Source: CAD feature listing. Evaluate the final solid. Frame: model axes, mm. Face numbers are marked on the shaded views. Give positions to 0.01 mm unless a question says otherwise; leave off trailing zeros. Order: outer loops, then holes, each group sorted by start corner. A loop starts at its lowest first (then second) coordinate and runs counter-clockwise, first axis right, second up. Notation, with made-up numbers: M 4,-1 L 57,-1 A18 ccw 57,16 Z; hole C -32.5,-30 d1. An arc over 180 degrees is marked long. Return JSON: item names as keys, results as strings.
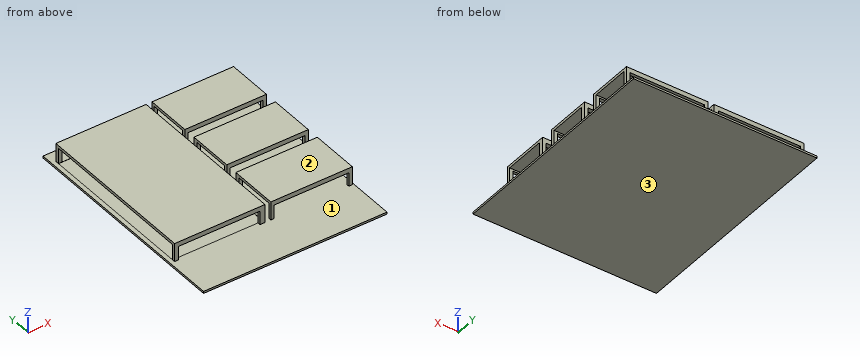
from build123d import *

# Parameters (mm, degrees)
SKETCH1_W               = 180
SKETCH1_H               = 220
BASE_DEPTH              = 2
SKETCH2_W               = 88.607017387
SKETCH2_H               = 162.747582956
SKETCH2_W_2             = 80
SKETCH2_H_2             = 45
SKETCH2_H_3             = 47.956874403
BOARDS_DEPTH            = 20
CUT_EXTRUDE1_DEPTH      = 285.956136976
CUT_EXTRUDE1_DEPTH_BACK = 285.956136976
SKETCH3_W               = 80.16842423
SKETCH3_H               = 13.497664936
SKETCH3_W_2             = 73.29684501
SKETCH4_W               = 15.397369521
SKETCH4_H               = 156.425076719
CUT_EXTRUDE2_DEPTH      = 88.607017387
SKETCH5_W               = 15.24584824
SKETCH5_H               = 38.4651821
SKETCH5_H_2             = 37.437486396
SKETCH5_H_3             = 40.814200855
CUT_EXTRUDE3_DEPTH      = 80


with BuildPart() as part:
    # Sketch1 → Base (new body)
    with BuildSketch(Plane.XY):
        with Locations((90, 110)):
            Rectangle(SKETCH1_W, SKETCH1_H)
    extrude(amount=BASE_DEPTH)

    # Sketch2 → Boards (add)
    with BuildSketch(Plane.XY):
        with Locations((48.5089102, 126.904245713)):
            Rectangle(SKETCH2_W, SKETCH2_H)
        with Locations((138.596199401, 185.778037191)):
            Rectangle(SKETCH2_W_2, SKETCH2_H_2)
        with Locations((138.596199401, 128.382682915)):
            Rectangle(SKETCH2_W_2, SKETCH2_H_2)
        with Locations((138.596199401, 69.508891437)):
            Rectangle(SKETCH2_W_2, SKETCH2_H_3)
    extrude(amount=BOARDS_DEPTH)

    # Sketch3 → Cut-Extrude1 (cut, two sides: drawn at the far end of the back side and taken through both)
    with BuildSketch(Plane(origin=(0, 0, 0), x_dir=(1, 0, 0), z_dir=(0, 1, 0)).offset(-CUT_EXTRUDE1_DEPTH_BACK)):
        with Locations((48.029472021, -8.748832468)):
            Rectangle(SKETCH3_W, SKETCH3_H)
        with Locations((138.50526508, -8.748832468)):
            Rectangle(SKETCH3_W_2, SKETCH3_H)
    extrude(amount=CUT_EXTRUDE1_DEPTH + CUT_EXTRUDE1_DEPTH_BACK, mode=Mode.SUBTRACT)

    # Sketch4 → Cut-Extrude2 (cut)
    with BuildSketch(Plane(origin=(92.812418893, 0, 0), x_dir=(0, 0, -1), z_dir=(1, 0, 0))):
        with Locations((-9.547163479, 126.516271725)):
            Rectangle(SKETCH4_W, SKETCH4_H)
    extrude(amount=-CUT_EXTRUDE2_DEPTH, mode=Mode.SUBTRACT)

    # Sketch5 → Cut-Extrude3 (cut)
    with BuildSketch(Plane(origin=(178.596199401, 0, 0), x_dir=(0, 0, -1), z_dir=(1, 0, 0))):
        with Locations((-9.62292412, 186.029564078)):
            Rectangle(SKETCH5_W, SKETCH5_H)
        with Locations((-9.62292412, 127.817943074)):
            Rectangle(SKETCH5_W, SKETCH5_H_2)
        with Locations((-9.62292412, 68.578626366)):
            Rectangle(SKETCH5_W, SKETCH5_H_3)
    extrude(amount=-CUT_EXTRUDE3_DEPTH, mode=Mode.SUBTRACT)


solid = part.part
1. Section query B-B (y = 139). Return loops of the section in (x, z), then the cut area to 3 significant figures.
Evaluation:
{"outline": "M 0,0 L 180,0 L 180,2 L 92.81,2 L 92.81,1.85 L 4.21,1.85 L 4.21,2 L 0,2 Z; M 4.21,17.25 L 92.81,17.25 L 92.81,20 L 4.21,20 Z; M 98.6,17.25 L 178.6,17.25 L 178.6,20 L 98.6,20 Z", "area": "811 mm^2"}
2. Section query A-A (x = 154.5). Return loops of the section in (y, z).
Evaluation:
{"outline": "M 0,0 L 220,0 L 220,2 L 0,2 Z; M 45.53,15.5 L 48.17,15.5 L 48.17,17.25 L 88.99,17.25 L 88.99,15.5 L 93.49,15.5 L 93.49,20 L 45.53,20 Z; M 105.88,15.5 L 109.1,15.5 L 109.1,17.25 L 146.54,17.25 L 146.54,15.5 L 150.88,15.5 L 150.88,20 L 105.88,20 Z; M 163.28,15.5 L 166.8,15.5 L 166.8,17.25 L 205.26,17.25 L 205.26,15.5 L 208.28,15.5 L 208.28,20 L 163.28,20 Z"}
3. Ray query, probe 1 along Y at (x, z) = (147, 17.75); probe 2 along Y at (x, z) = (90.5, 13.75); probe 3 along Z at (x, y) = (152.5, 127.5). Return the intervals inside material, ascending.
Evaluation:
{"probe 1": "y = 45.53 to 93.49, 105.88 to 150.88, 163.28 to 208.28", "probe 2": "y = 45.53 to 48.3, 204.73 to 208.28", "probe 3": "z = 0 to 2, 17.25 to 20"}
4. Section query D-D (x = 58). Return loops of the section in (y, z), then the cut area to 3 significant figures.
Evaluation:
{"outline": "M 0,0 L 220,0 L 220,2 L 204.73,2 L 204.73,1.85 L 48.3,1.85 L 48.3,2 L 0,2 Z; M 45.53,15.5 L 48.3,15.5 L 48.3,17.25 L 204.73,17.25 L 204.73,15.5 L 208.28,15.5 L 208.28,20 L 45.53,20 Z", "area": "876 mm^2"}
5. Section query C-C (y = 96.5). Return loops of the section in (x, z), then the cut area to 3 significant figures.
Evaluation:
{"outline": "M 0,0 L 180,0 L 180,2 L 92.81,2 L 92.81,1.85 L 4.21,1.85 L 4.21,2 L 0,2 Z; M 4.21,17.25 L 92.81,17.25 L 92.81,20 L 4.21,20 Z", "area": "591 mm^2"}
6. Draft query along Z for the marked faces 1, 2 and 3. Return one class per face: pulls with the +Z half, pulls with the -Z half, needs draft (parallel to the pull), parting line crosses it, or undercut.
Evaluation:
{"face 1": "undercut", "face 2": "pulls with the +Z half", "face 3": "pulls with the -Z half"}
7. First-contact query: pin 1 (1.3 mm diameter, centred on y = 148, z = 12, fed in from -X); pin 2 (0.9 mm diameter, centred on y = 206.5, z = 6, fed in from +X); pin 3 (2 mm diameter, centred on y = 47, z = 6.5, fed in from -X). Flat tips, straight axial feed; report the tip coordinate or a pass-through.
Evaluation:
{"pin 1": "stops at x = 98.6", "pin 2": "stops at x = 178.6", "pin 3": "stops at x = 4.21"}
